Geometry: final body of the model. Coordinates: model frame, mm. Face numbers are marked on the shaded views. A direction names the side the tool comes from. Give positions to 0.01 mm unless a question says otherwise; leave off trailing zeros. Order: outer loops, then holes, each group sorted by start corner. A loop starts at its lowest first (then second) coordinate and runs counter-clockwise, first axis right, second up. Notation, with made-up numbers: (55, 7) - (98, 7) arc R17 cw to (98, 37) - close; hole circle Ø9 at (-24.75, -10). An arc over 180 degrees is marked (long way). Write item = value, one per line. Start each with the question number.
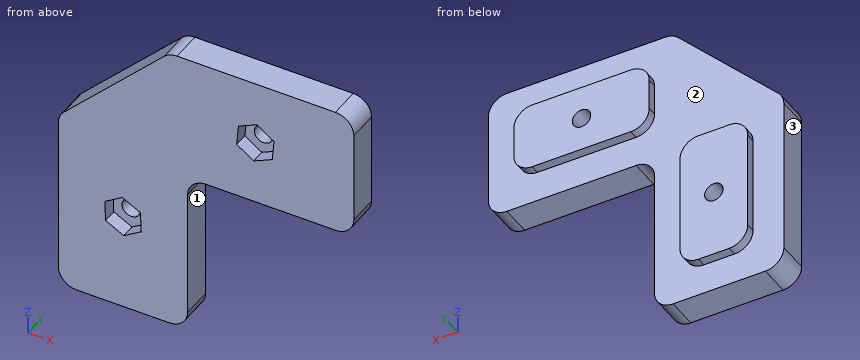
from build123d import *

# Parameters (mm, degrees)
SALIENTE_EXTRUIR1_DEPTH   = 1.5
SALIENTE_EXTRUIR1_2_DEPTH = 1.5
SALIENTE_EXTRUIR2_DEPTH   = 5
CROQUIS3_R                = 1.5
CORTAR_EXTRUIR1_DEPTH     = 45
CORTAR_EXTRUIR2_DEPTH     = 2.3
CROQUIS5_R                = 1.5
CORTAR_EXTRUIR3_DEPTH     = 42.3
CORTAR_EXTRUIR4_DEPTH     = 2.3


with BuildPart() as part:
    # Croquis1 → Saliente-Extruir1 (new body)
    with BuildSketch(Plane(origin=(0, 0, 0), x_dir=(1, 0, 0), z_dir=(0, 1, 0))):
        with BuildLine():
            Line((3, 38), (8, 38))
            ThreePointArc((8, 38), (10.121320344, 37.121320344), (11, 35))
            Line((11, 35), (11, 19))
            ThreePointArc((11, 19), (10.121320344, 16.878679656), (8, 16))
            Line((8, 16), (3, 16))
            ThreePointArc((3, 16), (0.878679656, 16.878679656), (0, 19))
            Line((0, 19), (0, 35))
            ThreePointArc((0, 35), (0.878679656, 37.121320344), (3, 38))
        make_face()
    extrude(amount=SALIENTE_EXTRUIR1_DEPTH)



with BuildPart() as body_2:
    # Croquis1 → Saliente-Extruir1 2 (new body)
    with BuildSketch(Plane(origin=(0, 0, 0), x_dir=(1, 0, 0), z_dir=(0, 1, 0))):
        with BuildLine():
            Line((19, 11), (35, 11))
            ThreePointArc((35, 11), (37.121320344, 10.121320344), (38, 8))
            Line((38, 8), (38, 3))
            ThreePointArc((38, 3), (37.121320344, 0.878679656), (35, 0))
            Line((35, 0), (19, 0))
            ThreePointArc((19, 0), (16.878679656, 0.878679656), (16, 3))
            Line((16, 3), (16, 8))
            ThreePointArc((16, 8), (16.878679656, 10.121320344), (19, 11))
        make_face()
    extrude(amount=SALIENTE_EXTRUIR1_2_DEPTH)


with BuildPart() as part_1:
    add(part.part)

    add(body_2.part)  # Saliente-Extruir2 merges body 2
    # Croquis2 → Saliente-Extruir2 (add)
    with BuildSketch(Plane(origin=(0, 0, 0), x_dir=(1, 0, 0), z_dir=(0, 1, 0))):
        with BuildLine():
            Line((-2, 43), (13, 43))
            ThreePointArc((13, 43), (15.121320344, 42.121320344), (16, 40))
            Line((16, 40), (16, 19))
            ThreePointArc((16, 19), (16.878679656, 16.878679656), (19, 16))
            Line((19, 16), (40, 16))
            ThreePointArc((40, 16), (42.121320344, 15.121320344), (43, 13))
            Line((43, 13), (43, -2))
            ThreePointArc((43, -2), (42.121320344, -4.121320344), (40, -5))
            Line((40, -5), (14.269081713, -5))
            ThreePointArc((14.269081713, -5), (13.121031415, -4.771638598), (12.147761369, -4.121320344))
            Line((12.147761369, -4.121320344), (-4.121320344, 12.147761369))
            ThreePointArc((-4.121320344, 12.147761369), (-4.771638598, 13.121031415), (-5, 14.269081713))
            Line((-5, 14.269081713), (-5, 40))
            ThreePointArc((-5, 40), (-4.121320344, 42.121320344), (-2, 43))
        make_face()
    extrude(amount=-SALIENTE_EXTRUIR2_DEPTH)

    # Croquis3 → Cortar-Extruir1 (cut)
    with BuildSketch(Plane(origin=(0, 1.5, 0), x_dir=(1, 0, 0), z_dir=(0, 1, 0))):
        with Locations(Location((5.5, 27, 0), (0, 0, 270))):
            Circle(CROQUIS3_R)
    extrude(amount=-CORTAR_EXTRUIR1_DEPTH, mode=Mode.SUBTRACT)

    # Croquis4 → Cortar-Extruir2 (cut)
    with BuildSketch(Plane.XZ.offset(5)):
        Polygon((2.669346369, -28.789059349), (5.634044029, -30.345947628), (8.464697661, -28.556888279), (8.330653631, -25.210940651), (5.365955971, -23.654052372), (2.535302339, -25.443111721), align=None)
    extrude(amount=-CORTAR_EXTRUIR2_DEPTH, mode=Mode.SUBTRACT)

    # Croquis5 → Cortar-Extruir3 (cut)
    with BuildSketch(Plane(origin=(0, 1.5, 0), x_dir=(1, 0, 0), z_dir=(0, 1, 0))):
        with Locations(Location((27, 5.5, 0), (0, 0, 270))):
            Circle(CROQUIS5_R)
    extrude(amount=-CORTAR_EXTRUIR3_DEPTH, mode=Mode.SUBTRACT)

    # Croquis8 → Cortar-Extruir4 (cut)
    with BuildSketch(Plane.XZ.offset(5)):
        Polygon((24.250581209, -3.588448368), (23.96983833, -6.925290703), (26.719257122, -8.836842335), (29.749418791, -7.411551632), (30.03016167, -4.074709297), (27.280742878, -2.163157665), align=None)
    extrude(amount=-CORTAR_EXTRUIR4_DEPTH, mode=Mode.SUBTRACT)


solid = part_1.part
Q1. Section D-D, the plane z = -27. Return the cut outline in (x, y), then the cut area to 3 significant figures.
Q2. Contact query for flat-ended pins moving along their axis: pin 1 (0.8 mm diameter, centred on y = 0.5, z = -5, fed in from -X); pin 2 (6 mm diameter, centred on x = 17.5, z = -31, fed in from +Y); pin 3 (1.5 mm diameter, centred on x = 29.5, y = -3.5, fed in from -Z); pin 4 (2.5 mm diameter, centred on x = 5.5, z = -27, fed in from -Y) (1 decimal). Output: stop coordinate, or through.
Q3. Section C-C, the plane x = 33.5. Return the cut outline in (y, z), then the cut area to 4 significant figures.
Q4. Material intervals for line 1 along X through (y, z) = (-1.6, -27); line 2 along X through (y, z) = (-0.05, -5.5); line 3 along Y through (x, z) = (34, -13), sorted ascending. Write a range as from..to.
Q5. Section B-B, the plane z = -5.5. Return the cut outline in (x, y), then the cut area to 3 significant figures.
Q6. Set-up query: the marked faces 1, 2 and 3. Return all of +Z, -Z, +X, -X, +Y, -Y with unobstructed straight access to the full face (end or side cutting, diameter ignored); none if empty.
Q7. Section A-A, the plane y = -3.75. Return the cut outline in (x, z).
The answers:
q1.outline = (-5, -5) - (2.6, -5) - (2.6, -2.7) - (4, -2.7) - (4, 1.5) - (0, 1.5) - (0, 0) - (-5, 0) - close; (7, -2.7) - (8.4, -2.7) - (8.4, -5) - (16, -5) - (16, 0) - (11, 0) - (11, 1.5) - (7, 1.5) - close
q1.area = 95.5 mm²
q2.pin_1 = 16
q2.pin_2 = 0
q2.pin_3 = -16
q2.pin_4 = through
q3.outline = (-5, -16) - (0, -16) - (0, -11) - (1.5, -11) - (1.5, 0) - (0, 0) - (0, 5) - (-5, 5) - close
q3.area = 121.5 mm²
q4.line_1 = -5..4, 7..16
q4.line_2 = 2.53..25.5, 28.5..43
q4.line_3 = -5..0
q5.outline = (2.53, -5) - (24.09, -5) - (24.09, -2.7) - (25.5, -2.7) - (25.5, 1.5) - (16, 1.5) - (16, 0) - (2.53, 0) - close; (28.5, -2.7) - (29.91, -2.7) - (29.91, -5) - (43, -5) - (43, 0) - (38, 0) - (38, 1.5) - (28.5, 1.5) - close
q5.area = 209 mm²
q6.face_1 = -Z, +X, +Y, -Y
q6.face_2 = +Y
q6.face_3 = +Z, -Z, -X, +Y, -Y
q7.outline = (-5, -40) arc R3 ccw to (-2, -43) - (13, -43) arc R3 ccw to (16, -40) - (16, -19) arc R3 cw to (19, -16) - (40, -16) arc R3 ccw to (43, -13) - (43, 2) arc R3 ccw to (40, 5) - (14.27, 5) arc R3 ccw to (12.15, 4.12) - (-4.12, -12.15) arc R3 ccw to (-5, -14.27) - close; hole (2.54, -25.44) - (2.67, -28.79) - (5.63, -30.35) - (8.46, -28.56) - (8.33, -25.21) - (5.37, -23.65) - close; hole (23.97, -6.93) - (26.72, -8.84) - (29.75, -7.41) - (30.03, -4.07) - (27.28, -2.16) - (24.25, -3.59) - close
